from build123d import *

# Parameters (mm, degrees)
F0_W     = 159
F0_H     = 129
F1_DEPTH = 60
F2_R     = 12
F2_R_2   = 9
F3_DEPTH = 5.5
F4_R     = 5
F6_D     = 3.505
F7_SIZE  = 1


with BuildPart() as f1:
    # F0 (on Front) → F1 (new body)
    with BuildSketch(Plane.XZ):
        with Locations((5.110869, -2.757801)):
            Rectangle(F0_W, F0_H)
    extrude(amount=F1_DEPTH)

    # F2 (on face) → F3 (join)
    with BuildSketch(Plane.XZ.offset(60)):
        with Locations((-61.389131, 29.242199)):
            Circle(F2_R)
        with Locations((-61.389131, 29.242199)):
            Circle(F2_R_2, mode=Mode.SUBTRACT)
        with Locations((-61.389131, -34.757801)):
            Circle(F2_R)
        with Locations((-61.389131, -34.757801)):
            Circle(F2_R_2, mode=Mode.SUBTRACT)
    extrude(amount=F3_DEPTH)

    # F4
    f4_edges = [f1.edges().sort_by_distance(p)[0] for p in [
        (84.610869, -30, -67.257801),
        (84.610869, -30, 61.742199),
        (-74.389131, -30, 61.742199),
        (-74.389131, -30, -67.257801),
    ]]
    fillet(f4_edges, radius=F4_R)

    # F6 (through all)
    with Locations(Plane.XZ.offset(60)):
        with Locations((-38.889131, 49.742199), (66.110869, 49.742199), (-38.889131, -55.257801), (66.110869, -55.257801)):
            Hole(F6_D / 2)

    # F7
    f7_edges = [f1.edges().sort_by_distance(p)[0] for p in [
        (-73.389131, -65.5, 29.242199),
        (-73.389131, -65.5, -34.757801),
    ]]
    chamfer(f7_edges, length=F7_SIZE)


solid = f1.part
Build history of the part. All positions in model axes, mm. A direction names the side the tool comes from. Coordinates: 2 decimals unless noted, no trailing zeros. Order: outer loops, then holes, each group sorted by start corner. A loop starts at its lowest first (then second) coordinate and runs counter-clockwise, first axis right, second up. Notation, with made-up numbers: (53.25, 42) - (92.25, 42) arc R18 cw to (92.25, 57) - close; hole circle Ø3 at (88, 61.5). An arc over 180 degrees is marked (long way). Write each question's results on one line, items separated by ' | '. Start each with the question number.
Item 1: Flat gauge pin, fed straight in: pin 1 (8 mm diameter, centred on x = -34, z = 8.5, fed in from -Y). Where does the tip first touch, or does it go through?
Item 2: Mould opens along Z. For faces 1 (the face through (-53.075, -62.712, -38.205)), 2 (the face through (-72.963, -30.42, -65.754)), 3 (the face through (4, 0, -2)), 4 (the face through (83.107, -30.42, 60.316)) say: released by +Z, released by -Z, zero draft, split by the parting line, or undercut.
Item 3: Band-saw the part on A-A on z = -48.5. Write the cut outline in (x, y).
Item 4: Wall check: probe 1 along X at (y, z) = (-3, -55); probe 2 along Z at (x, y) = (64.5, -18.5); probe 3 along Y at (x, z) = (-12, 12). Give the ranges that are in metal, low to high. Write a range as [from, to].
Item 5: Tool access for faces 5 (the face through (-52.805, -62.712, 31.946)), 6 (the face through (4, -30, -67.258)): list every direction of +Z, -Z, +X, -X, +Y, -Y with a clear straight run to the whole face (end or side of a thin tool).
Item 6: Band-saw the part on B-B on x = 28.5. Write the cut outline in (y, z).
Numbers:
1) pin 1: y = -60
2) face 1: undercut | face 2: released by -Z | face 3: zero draft | face 4: released by +Z
3) outline: (-74.39, -60) - (84.61, -60) - (84.61, 0) - (-74.39, 0) - close
4) probe 1: [-74.39, -40.62], [-37.16, 64.38], [67.84, 84.61] | probe 2: [-67.26, -55.95], [-54.57, 49.05], [50.43, 61.74] | probe 3: [-60, 0]
5) face 5: -Y | face 6: -Z, +X, -X, +Y, -Y
6) outline: (-60, -67.26) - (0, -67.26) - (0, 61.74) - (-60, 61.74) - close
